Work out the finished part from the listing and answer in its coordinate system (mm). A direction names the side the tool comes from. Round coordinates to 2 decimals unless told otherwise and drop trailing zeros. Order: outer loops, then holes, each group sorted by start corner. A loop starts at its lowest first (then second) coordinate and runs counter-clockwise, first axis right, second up. Notation, with made-up numbers: (17, 2.5) -> (66, 2.5) arc R19 ccw to (66, 29.5) -> close; hole circle Ø4 at (-29, 5). An arc over 180 degrees is marked (long way). Use a Markdown table: item, result. Add a question column.
Item 1: Flat-ended cylindrical pins translate along their axes: P1, Ø2, axis at x = 2, z = 139, coming from the +Y side; P2, Ø2, axis at x = 1.5, z = 3.5, coming from the -Y side. Find the tip coordinate at first contact, or state that the pin passes through.
Item 2: A cutting plane is placed at A-A, the plane y = 60. Determine the outline of the cut face in (x, z), plus the area to 3 significant figures.
Item 3: For a pull along Z with two mould halves and no side action, classify faces 1 (the flat face through (1.972, -31.508, -8.156)), 2 (the flat face through (2, 78, 149)), 3 (the flat face through (0, 28, 30)) as +Z half, -Z half, draft (parallel to the pull), parting line (faces both ways), or undercut.
Item 4: A cutting plane is placed at C-C, the plane x = 0.7. Give the number of separate pieces and of enclosed holes in the cut face, plus the area to 3 significant figures.
Item 5: A tool of negligible diameter and unlimited length cuts with its end or side. For faces 4 (the flat face through (2.028, -18.975, 97.537)), 5 (the flat face through (4, 28, 30)), from which of +Z, -Z, +X, -X, +Y, -Y can it reach the whole face along a straight path? Write none if from no direction.
Item 6: A cutting plane is placed at B-B, the plane z = -30.5. Determine the outline of the cut face in (x, y).
Item 7: Find the intervals of material crossed by L1, parallel to Z at x = 2.55, y = 8.5; L2, parallel to Y at x = 3.5, z = -50; L3, parallel to Z at x = 0.4, y = 19, in increasing order. Write a range as [from, to].
from build123d import *

# Parameters (mm, degrees)
F1_DEPTH  = 4
F2_R      = 4
F3_W      = 4
F3_H      = 10
F4_DEPTH  = 4
F5_W      = 4
F5_H      = 10
F5_W_2    = 10
F5_H_2    = 4
F6_DEPTH  = 4
F8_DEPTH  = 4
F9_R      = 4
F10_W     = 10
F10_H     = 4
F10_W_2   = 4
F10_H_2   = 10
F11_DEPTH = 25
F12_R     = 4


with BuildPart() as f1:
    # F0 (on Right) → F1 (new body)
    with BuildSketch(Plane.YZ):
        Polygon((0, 92.128), (0, 0), (-63.825185854, -16.522066811), (-63.825185854, -102.781066811), (87.919814146, -102.781066811), (87.919814146, 92.128), align=None)
        Polygon((-52.2425177801, -17.65557521), (-42.5616207767, -15.149535863), (-41.5592050378, -19.0218946644), (-51.2401020413, -21.5279340114), align=None, mode=Mode.SUBTRACT)
        Polygon((-32.8807237732, -12.643496516), (-23.1998267698, -10.1374571689), (-22.197411031, -14.0098159703), (-31.8783080344, -16.5158553174), align=None, mode=Mode.SUBTRACT)
        Polygon((-13.5189297663, -7.6314178219), (-3.8380327629, -5.1253784749), (-2.8356170241, -8.9977372763), (-12.5165140275, -11.5037766233), align=None, mode=Mode.SUBTRACT)
    extrude(amount=F1_DEPTH)

    # F2
    f2_edges = [f1.edges().sort_by_distance(p)[0] for p in [
        (2, -63.825186, -16.522067),
    ]]
    fillet(f2_edges, radius=F2_R)

    # F3 (on face) → F4 (cut)
    with BuildSketch(Plane.YZ.offset(4)):
        with Locations((9.0024157388, 86.1276411986)):
            Rectangle(F3_W, F3_H)
        with Locations((9.0024157388, 66.1276411986)):
            Rectangle(F3_W, F3_H)
        with Locations((9.0024157388, 46.1276411986)):
            Rectangle(F3_W, F3_H)
        with Locations((9.0024157388, 26.1276411986)):
            Rectangle(F3_W, F3_H)
        with Locations((9.0024157388, 6.1276411986)):
            Rectangle(F3_W, F3_H)
    extrude(amount=-F4_DEPTH, mode=Mode.SUBTRACT)

    # F5 (on face) → F6 (cut)
    with BuildSketch(Plane.YZ.offset(4)):
        with Locations((-54.080550543, -32.7809536849)):
            Rectangle(F5_W, F5_H)
        with Locations((-54.080550543, -52.7809536849)):
            Rectangle(F5_W, F5_H)
        with Locations((-54.080550543, -72.7809536849)):
            Rectangle(F5_W, F5_H)
        with Locations((-54.080550543, -92.7809536849)):
            Rectangle(F5_W, F5_H)
        with Locations((-2.080550543, -100.781066811)):
            Rectangle(F5_W_2, F5_H_2)
        with Locations((17.919449457, -100.781066811)):
            Rectangle(F5_W_2, F5_H_2)
        with Locations((37.919449457, -100.781066811)):
            Rectangle(F5_W_2, F5_H_2)
        with Locations((-22.080550543, -100.781066811)):
            Rectangle(F5_W_2, F5_H_2)
        with Locations((-42.080550543, -100.781066811)):
            Rectangle(F5_W_2, F5_H_2)
        with Locations((57.919449457, -100.781066811)):
            Rectangle(F5_W_2, F5_H_2)
        with Locations((77.919449457, -100.781066811)):
            Rectangle(F5_W_2, F5_H_2)
    extrude(amount=-F6_DEPTH, mode=Mode.SUBTRACT)

    # F7 (on face) → F8 (join)
    with BuildSketch(Plane.YZ.offset(4)):
        Polygon((-37.5059572495, 102.8192660989), (0, 92.128), (87.919814146, 92.128), (87.919814146, 159.5652660989), (-37.5059572495, 159.5652660989), align=None)
    extrude(amount=-F8_DEPTH)

    # F9
    f9_edges = [f1.edges().sort_by_distance(p)[0] for p in [
        (2, -37.505957, 159.565266),
        (2, 87.919814, 159.565266),
        (2, -37.505957, 102.819266),
    ]]
    fillet(f9_edges, radius=F9_R)

    # F10 (on face) → F11 (cut)
    with BuildSketch(Plane(origin=(0, 0, 0), x_dir=(0, -1, 0), z_dir=(-1, 0, 0))):
        Polygon((-1.0965401127, 101.9704806816), (0, 98.1237158355), (9.6169121153, 100.8650661173), (8.5203720026, 104.7118309634), align=None)
        with Locations((22.5626522907, 153.5652066678)):
            Rectangle(F10_W, F10_H)
        with Locations((30.5626522907, 141.5652066678)):
            Rectangle(F10_W_2, F10_H_2)
        with Locations((30.5626522907, 121.5652066678)):
            Rectangle(F10_W_2, F10_H_2)
        Polygon((18.1372841178, 107.4531812452), (19.2338242305, 103.6064163991), (28.8507363458, 106.3477666808), (27.7541962331, 110.1945315269), align=None)
        with Locations((2.5626522907, 153.5652066678)):
            Rectangle(F10_W, F10_H)
        with Locations((-17.4373477093, 153.5652066678)):
            Rectangle(F10_W, F10_H)
        with Locations((-37.4373477093, 153.5652066678)):
            Rectangle(F10_W, F10_H)
        Polygon((-80.7050293604, 146.2975250167), (-71.4373477093, 155.5652066678), (-67.4372882782, 159.5652660989), (-87.919814146, 159.5652660989), (-87.919814146, 139.0827402311), align=None)
        with Locations((-57.4373477093, 153.5652066678)):
            Rectangle(F10_W, F10_H)
    extrude(amount=-F11_DEPTH, mode=Mode.SUBTRACT)

    # F12
    f12_edges = [f1.edges().sort_by_distance(p)[0] for p in [
        (2, 67.437288, 159.565266),
        (2, 87.919814, 139.08274),
        (2, 0, 92.128),
        (2, 0, 0),
    ]]
    fillet(f12_edges, radius=F12_R)


solid = f1.part
Reported:
| question | item | result |
|---|---|---|
| 1 | P1 | y = 87.88 |
| 1 | P2 | y = -0.04 |
| 2 | outline | (0, -98.78) -> (4, -98.78) -> (4, 151.57) -> (0, 151.57) -> close; (0, 155.57) -> (4, 155.57) -> (4, 159.57) -> (0, 159.57) -> close |
| 2 | area | 1,020 mm² |
| 3 | face 1 | undercut |
| 3 | face 2 | +Z half |
| 3 | face 3 | draft |
| 4 | separate pieces | 1 |
| 4 | enclosed holes | 21 |
| 4 | area | 30,100 mm² |
| 5 | face 4 | +X, -X, -Y |
| 5 | face 5 | +Z, -Z, +X, +Y, -Y |
| 6 | outline | (0, -63.83) -> (4, -63.83) -> (4, -56.08) -> (0, -56.08) -> close; (0, -52.08) -> (4, -52.08) -> (4, 87.92) -> (0, 87.92) -> close |
| 7 | L1 | [-102.78, 1.13], [11.13, 21.13], [31.13, 41.13], [51.13, 61.13], [71.13, 81.13], [91.13, 159.57] |
| 7 | L2 | [-63.83, -56.08], [-52.08, 87.92] |
| 7 | L3 | [-98.78, 151.57], [155.57, 159.57] |
